The model under review builds one solid part; all positions refer to its coordinate system, in mm. A direction names the side the tool comes from. Round coordinates to 2 decimals unless told otherwise and drop trailing zeros. Loops run counter-clockwise (first coordinate to the right, second up) from the corner with the lowest first, then second, coordinate; pieces in that order, holes last. Notation, with made-up numbers: M 43,-3 L 101,-3 A21 ccw 101,2 Z; hole C 34,67.25 d11. An arc over 180 degrees is marked long. Return JSON: item names as keys, results as strings. Group by question number.
Q1. Consider section B-B (x = 90). State the section outline as (y, z) points, and give its area (3 significant figures).
Q2. Consider section A-A (z = -45). State the section outline as (x, y) points.
Q3. To check wall thickness, follow line 1 along X through (y, z) = (-4.25, 88.9); line 2 along Z through (x, y) = (180, -9); line 3 along X through (y, z) = (-11, -88.9). State the ranges of each line that lie inside material, in increasing order.
Q4. Consider section C-C (y = -8.75). Count the separate pieces of the cut face and the enclosed holes in it, and give its area (3 significant figures).
Q5. Draft analysis for pull direction Z (two halves, no side actions). For faces 1 (the face through (-228.6, -6, 1)), 2 (the face through (-3, -6, 101.6)), 3 (the face through (198.41, -6.26, 39.2)), state which applies: pulls with the +Z half, pulls with the -Z half, needs draft (parallel to the pull), parting line crosses it, or undercut.
Q6. Clearance check with a flat-ended pin moving along its axis: pin 1 Ø3.5 at (x, z) = (1, -90.5) entering from +Y. State where the tip first meets the part, or that it passes through.
Q7. Consider section D-D (z = 51.5). State the section outline as (x, y) points.
Q8. For faces 4 (the face through (-212, -6.35, 89)), 5 (the face through (-3, 0, -1)), list the 3-axis set-ups (+Z, -Z, +X, -X, +Y, -Y) from which the entire face can be reached by the end or side of a thin tool; tool diameter is ignored.
from build123d import *

# Parameters (mm, degrees)
SKETCH1_W                                        = 457.2
SKETCH1_H                                        = 203.2
BOSS_EXTRUDE1_DEPTH                              = 12.7
CUT_EXTRUDE1_REACH                               = 14.7
SKETCH2_R                                        = 19.304
CBORE_FOR_1_4_SOCKET_HEAD_CAP_SCREW1_D           = 6.7564
CBORE_FOR_1_4_SOCKET_HEAD_CAP_SCREW1_DEPTH       = 12.7
CBORE_FOR_1_4_SOCKET_HEAD_CAP_SCREW1_CBORE_D     = 11.1125
CBORE_FOR_1_4_SOCKET_HEAD_CAP_SCREW1_CBORE_DEPTH = 6.35


with BuildPart() as part:
    # Sketch1 → Boss-Extrude1 (new body)
    with BuildSketch(Plane(origin=(0, 0, 0), x_dir=(1, 0, 0), z_dir=(0, 1, 0))):
        Rectangle(SKETCH1_W, SKETCH1_H)
    extrude(amount=-BOSS_EXTRUDE1_DEPTH)

    # Sketch2 → Cut-Extrude1 (cut, up to next)
    with BuildSketch(Plane(origin=(0, 0, 0), x_dir=(1, 0, 0), z_dir=(0, 1, 0)), mode=Mode.PRIVATE) as cut_extrude1_sk1:
        with Locations((-180, 45)):
            Circle(SKETCH2_R)
    cut_extrude1_tool1 = extrude(cut_extrude1_sk1.sketch, amount=-CUT_EXTRUDE1_REACH, mode=Mode.PRIVATE) & part.part
    add(cut_extrude1_tool1.solids().sort_by_distance((-180, 0, -45))[0], mode=Mode.SUBTRACT)
    # Sketch2 → Cut-Extrude1 (cut, up to next)
    with BuildSketch(Plane(origin=(0, 0, 0), x_dir=(1, 0, 0), z_dir=(0, 1, 0)), mode=Mode.PRIVATE) as cut_extrude1_sk2:
        with Locations((-90, 45)):
            Circle(SKETCH2_R)
    cut_extrude1_tool2 = extrude(cut_extrude1_sk2.sketch, amount=-CUT_EXTRUDE1_REACH, mode=Mode.PRIVATE) & part.part
    add(cut_extrude1_tool2.solids().sort_by_distance((-90, 0, -45))[0], mode=Mode.SUBTRACT)
    # Sketch2 → Cut-Extrude1 (cut, up to next)
    with BuildSketch(Plane(origin=(0, 0, 0), x_dir=(1, 0, 0), z_dir=(0, 1, 0)), mode=Mode.PRIVATE) as cut_extrude1_sk3:
        with Locations((0, 45)):
            Circle(SKETCH2_R)
    cut_extrude1_tool3 = extrude(cut_extrude1_sk3.sketch, amount=-CUT_EXTRUDE1_REACH, mode=Mode.PRIVATE) & part.part
    add(cut_extrude1_tool3.solids().sort_by_distance((0, 0, -45))[0], mode=Mode.SUBTRACT)
    # Sketch2 → Cut-Extrude1 (cut, up to next)
    with BuildSketch(Plane(origin=(0, 0, 0), x_dir=(1, 0, 0), z_dir=(0, 1, 0)), mode=Mode.PRIVATE) as cut_extrude1_sk4:
        with Locations((-180, -45)):
            Circle(SKETCH2_R)
    cut_extrude1_tool4 = extrude(cut_extrude1_sk4.sketch, amount=-CUT_EXTRUDE1_REACH, mode=Mode.PRIVATE) & part.part
    add(cut_extrude1_tool4.solids().sort_by_distance((-180, 0, 45))[0], mode=Mode.SUBTRACT)
    # Sketch2 → Cut-Extrude1 (cut, up to next)
    with BuildSketch(Plane(origin=(0, 0, 0), x_dir=(1, 0, 0), z_dir=(0, 1, 0)), mode=Mode.PRIVATE) as cut_extrude1_sk5:
        with Locations((-90, -45)):
            Circle(SKETCH2_R)
    cut_extrude1_tool5 = extrude(cut_extrude1_sk5.sketch, amount=-CUT_EXTRUDE1_REACH, mode=Mode.PRIVATE) & part.part
    add(cut_extrude1_tool5.solids().sort_by_distance((-90, 0, 45))[0], mode=Mode.SUBTRACT)
    # Sketch2 → Cut-Extrude1 (cut, up to next)
    with BuildSketch(Plane(origin=(0, 0, 0), x_dir=(1, 0, 0), z_dir=(0, 1, 0)), mode=Mode.PRIVATE) as cut_extrude1_sk6:
        with Locations((0, -45)):
            Circle(SKETCH2_R)
    cut_extrude1_tool6 = extrude(cut_extrude1_sk6.sketch, amount=-CUT_EXTRUDE1_REACH, mode=Mode.PRIVATE) & part.part
    add(cut_extrude1_tool6.solids().sort_by_distance((0, 0, 45))[0], mode=Mode.SUBTRACT)
    # Sketch2 → Cut-Extrude1 (cut, up to next)
    with BuildSketch(Plane(origin=(0, 0, 0), x_dir=(1, 0, 0), z_dir=(0, 1, 0)), mode=Mode.PRIVATE) as cut_extrude1_sk7:
        with Locations((90, -45)):
            Circle(SKETCH2_R)
    cut_extrude1_tool7 = extrude(cut_extrude1_sk7.sketch, amount=-CUT_EXTRUDE1_REACH, mode=Mode.PRIVATE) & part.part
    add(cut_extrude1_tool7.solids().sort_by_distance((90, 0, 45))[0], mode=Mode.SUBTRACT)
    # Sketch2 → Cut-Extrude1 (cut, up to next)
    with BuildSketch(Plane(origin=(0, 0, 0), x_dir=(1, 0, 0), z_dir=(0, 1, 0)), mode=Mode.PRIVATE) as cut_extrude1_sk8:
        with Locations((90, 45)):
            Circle(SKETCH2_R)
    cut_extrude1_tool8 = extrude(cut_extrude1_sk8.sketch, amount=-CUT_EXTRUDE1_REACH, mode=Mode.PRIVATE) & part.part
    add(cut_extrude1_tool8.solids().sort_by_distance((90, 0, -45))[0], mode=Mode.SUBTRACT)
    # Sketch2 → Cut-Extrude1 (cut, up to next)
    with BuildSketch(Plane(origin=(0, 0, 0), x_dir=(1, 0, 0), z_dir=(0, 1, 0)), mode=Mode.PRIVATE) as cut_extrude1_sk9:
        with Locations((180, 45)):
            Circle(SKETCH2_R)
    cut_extrude1_tool9 = extrude(cut_extrude1_sk9.sketch, amount=-CUT_EXTRUDE1_REACH, mode=Mode.PRIVATE) & part.part
    add(cut_extrude1_tool9.solids().sort_by_distance((180, 0, -45))[0], mode=Mode.SUBTRACT)
    # Sketch2 → Cut-Extrude1 (cut, up to next)
    with BuildSketch(Plane(origin=(0, 0, 0), x_dir=(1, 0, 0), z_dir=(0, 1, 0)), mode=Mode.PRIVATE) as cut_extrude1_sk10:
        with Locations((180, -45)):
            Circle(SKETCH2_R)
    cut_extrude1_tool10 = extrude(cut_extrude1_sk10.sketch, amount=-CUT_EXTRUDE1_REACH, mode=Mode.PRIVATE) & part.part
    add(cut_extrude1_tool10.solids().sort_by_distance((180, 0, 45))[0], mode=Mode.SUBTRACT)

    # CBORE for 1/4 Socket Head Cap Screw1
    with Locations(Plane(origin=(0, 0, 0), x_dir=(1, 0, 0), z_dir=(0, 1, 0))):
        with Locations((-215.9, -88.9), (0, -88.9), (215.9, -88.9), (215.9, 88.9), (0, 88.9), (-215.9, 88.9)):
            CounterBoreHole(CBORE_FOR_1_4_SOCKET_HEAD_CAP_SCREW1_D / 2, CBORE_FOR_1_4_SOCKET_HEAD_CAP_SCREW1_CBORE_D / 2, CBORE_FOR_1_4_SOCKET_HEAD_CAP_SCREW1_CBORE_DEPTH, depth=CBORE_FOR_1_4_SOCKET_HEAD_CAP_SCREW1_DEPTH)


solid = part.part
Values:
{
 "1": {"outline": "M -12.7,-101.6 L 0,-101.6 L 0,-64.3 L -12.7,-64.3 Z; M -12.7,-25.7 L 0,-25.7 L 0,25.7 L -12.7,25.7 Z; M -12.7,64.3 L 0,64.3 L 0,101.6 L -12.7,101.6 Z", "area": "1,600 mm2"},
 "2": {"outline": "M -228.6,-12.7 L -199.3,-12.7 L -199.3,0 L -228.6,0 Z; M -160.7,-12.7 L -109.3,-12.7 L -109.3,0 L -160.7,0 Z; M -70.7,-12.7 L -19.3,-12.7 L -19.3,0 L -70.7,0 Z; M 19.3,-12.7 L 70.7,-12.7 L 70.7,0 L 19.3,0 Z; M 109.3,-12.7 L 160.7,-12.7 L 160.7,0 L 109.3,0 Z; M 199.3,-12.7 L 228.6,-12.7 L 228.6,0 L 199.3,0 Z"},
 "3": {"line 1": "x = -228.6 to -221.46, -210.34 to -5.56, 5.56 to 210.34, 221.46 to 228.6", "line 2": "z = -101.6 to -64.3, -25.7 to 25.7, 64.3 to 101.6", "line 3": "x = -228.6 to -219.28, -212.52 to -3.38, 3.38 to 212.52, 219.28 to 228.6"},
 "4": {"separate pieces": "1", "enclosed holes": "16", "area": "81,000 mm2"},
 "5": {"face 1": "needs draft", "face 2": "pulls with the +Z half", "face 3": "undercut"},
 "6": {"pin 1": "stops at y = -6.35"},
 "7": {"outline": "M -228.6,-12.7 L -198.18,-12.7 L -198.18,0 L -228.6,0 Z; M -161.82,-12.7 L -108.18,-12.7 L -108.18,0 L -161.82,0 Z; M -71.82,-12.7 L -18.18,-12.7 L -18.18,0 L -71.82,0 Z; M 18.18,-12.7 L 71.82,-12.7 L 71.82,0 L 18.18,0 Z; M 108.18,-12.7 L 161.82,-12.7 L 161.82,0 L 108.18,0 Z; M 198.18,-12.7 L 228.6,-12.7 L 228.6,0 L 198.18,0 Z"},
 "8": {"face 4": "+Y", "face 5": "+Z, -Z, +X, -X, +Y"}
}
